Read the model definition and answer for the solid it produces. Units are mm, in the model's axes. A direction names the side the tool comes from. Give positions to 0.01 mm unless a question says otherwise; leave off trailing zeros. Order: outer loops, then holes, each group sorted by start corner. A loop starts at its lowest first (then second) coordinate and runs counter-clockwise, first axis right, second up. Notation, with made-up numbers: (64, -2) - (69, -2) arc R20 ccw to (69, 6) - close; hole circle Ø11 at (-6.75, 4). An arc over 180 degrees is marked (long way). Return JSON: item names as keys, results as strings.
```python
from build123d import *

# Parameters (mm, degrees)
SKETCH1_R           = 1
SKETCH1_R_2         = 1.5
BOSS_EXTRUDE1_DEPTH = 3


with BuildPart() as part:
    # Sketch1 → Boss-Extrude1 (new body)
    with BuildSketch(Plane.XY):
        with BuildLine():
            Line((6.869152375, -4.974037541), (5.570032573, 2.020702591))
            ThreePointArc((5.570032573, 2.020702591), (0.408013999, 8.949092219), (-8.230691413, 9.096697763))
            ThreePointArc((-8.230691413, 9.096697763), (-8.247364434, 9.088837268), (-8.264022634, 9.080945414))
            ThreePointArc((-8.264022634, 9.080945414), (-13.168452035, 7.370807944), (-18.321933974, 6.723025711))
            Line((-18.321933974, 6.723025711), (-18.900934286, 6.723025711))
            Line((-18.900934286, 6.723025711), (-18.900934286, -5.309936566))
            Line((-18.900934286, -5.309936566), (-13.651422395, -5.309936566))
            ThreePointArc((-13.651422395, -5.309936566), (-12.600650913, -5.055458479), (-11.78274174, -4.34841931))
            ThreePointArc((-11.78274174, -4.34841931), (-8.658711941, -2.8651804), (-5.749146129, -4.734401261))
            ThreePointArc((-5.749146129, -4.734401261), (-3.178332185, -7.427632658), (0.410473142, -8.419124472))
            Line((0.410473142, -8.419124472), (4.004999648, -8.419124472))
            ThreePointArc((4.004999648, -8.419124472), (6.245088642, -7.368341001), (6.869152375, -4.974037541))
        make_face()
        with Locations((-0.216717362, -5.419124472)):
            Circle(SKETCH1_R, mode=Mode.SUBTRACT)
        with Locations((-1.756717362, 1.940875528)):
            Circle(SKETCH1_R_2, mode=Mode.SUBTRACT)
    extrude(amount=BOSS_EXTRUDE1_DEPTH)


solid = part.part
```
Q1. A cutting plane is placed at A-A (y = 1.25). Write down the section's boundary in (x, z), and give its area (3 significant figures).
Values:
{"outline": "(-18.9, 0) - (-3.09, 0) - (-3.09, 3) - (-18.9, 3) - close; (-0.43, 0) - (5.71, 0) - (5.71, 3) - (-0.43, 3) - close", "area": "65.9 mm²"}
Q2. Consider L1, parallel to Y at x = -1, z = 0.5; L2, parallel to X at y = 2, z = 2; L3, parallel to X at y = 1, z = 1.7. Determine where each line is inside the solid, lowest interval first.
Values:
{"L1": "y = -8.28 to -6.04, -4.8 to 0.65, 3.24 to 9.54", "L2": "x = -18.9 to -3.26, -0.26 to 5.57", "L3": "x = -18.9 to -2.92, -0.59 to 5.76"}
Q3. A cutting plane is placed at D-D (y = 4.75). Write down the section's boundary in (x, z), and give its area (3 significant figures).
Values:
{"outline": "(-18.9, 0) - (4.63, 0) - (4.63, 3) - (-18.9, 3) - close", "area": "70.6 mm²"}
Q4. A cutting plane is placed at B-B (x = -2). Write down the section's boundary in (y, z).
Values:
{"outline": "(-7.99, 0) - (0.46, 0) - (0.46, 3) - (-7.99, 3) - close; (3.42, 0) - (9.81, 0) - (9.81, 3) - (3.42, 3) - close"}
Q5. Determine the mould class of faces 3 (the flat face through (-6, 1, 0)), 4 (the cylindrical face through (-12.61, -5.06, 1.48)), 5 (the flat face through (6.23, -1.53, 1.48)), 6 (the flat face through (-18.901, 1, 1)) for opening direction X: released by +X, released by -X, zero draft, split by the parting line, or undercut.
Values:
{"face 3": "zero draft", "face 4": "undercut", "face 5": "released by +X", "face 6": "released by -X"}
Q6. A cutting plane is placed at C-C (z = 0.4). Write down the section's boundary in (x, y) (3 decimals).
Values:
{"outline": "(-18.901, -5.31) - (-13.651, -5.31) arc R2.297 ccw to (-11.783, -4.348) arc R3.56 cw to (-5.749, -4.734) arc R6.991 ccw to (0.41, -8.419) - (4.005, -8.419) arc R2.913 ccw to (6.869, -4.974) - (5.57, 2.021) arc R9.796 ccw to (-8.231, 9.097) arc R9.796 ccw to (-8.264, 9.081) arc R24.724 cw to (-18.322, 6.723) - (-18.901, 6.723) - close; hole circle Ø3 at (-1.757, 1.941); hole circle Ø2 at (-0.217, -5.419)"}
Q7. For faces 1 (the flat face through (2, -8.419, 1)), 2 (the flat face through (-16, -5.31, 1)), determine the directions among +Z, -Z, +X, -X, +Y, -Y from which every point of the face is accessible in a straight line to the end or side of a thin tool.
Values:
{"face 1": "+Z, -Z, +X, -X, -Y", "face 2": "+Z, -Z, -X, -Y"}
Q8. Given pin 1 (1 mm diameter, centred on x = 0.5, z = 2.5, fed in from +Y); pin 2 (0.9 mm diameter, centred on x = -15, z = 1, fed in from -Y); pin 3 (0.6 mm diameter, centred on x = -18.5, z = 1, fed in from +Y), each flat-ended and moving along its own axis, determine where each tip first touches the part or whether it passes through.
Values:
{"pin 1": "stops at y = 9.15", "pin 2": "stops at y = -5.31", "pin 3": "stops at y = 6.73"}
